Build history of the part. All positions in model axes, mm. Coordinates: 2 decimals unless noted, no trailing zeros. Order: outer loops, then holes, each group sorted by start corner. A loop starts at its lowest first (then second) coordinate and runs counter-clockwise, first axis right, second up. Notation, with made-up numbers: (86.25, 13) - (123.25, 13) arc R24 ccw to (123.25, 31) - close; hole circle Ø4 at (-11, 39). An arc over 180 degrees is marked (long way). Write each question's results on one line, items separated by ' | '.
from build123d import *

# Parameters (mm, degrees)
SKETCH1_W           = 63.5
SKETCH1_H           = 101.6
SKETCH1_R           = 20.955
SKETCH1_R_2         = 3.175
BOSS_EXTRUDE1_DEPTH = 4.7625
CHAMFER1_SIZE       = 3.8862
CHAMFER1_SIZE2      = 3.378222121


with BuildPart() as part:
    # Sketch1 → Boss-Extrude1 (new body)
    with BuildSketch(Plane(origin=(0, 0, 0), x_dir=(1, 0, 0), z_dir=(0, 1, 0))):
        with Locations((31.75, 50.8)):
            Rectangle(SKETCH1_W, SKETCH1_H)
        with Locations((31.75, 50.8)):
            Circle(SKETCH1_R, mode=Mode.SUBTRACT)
        with Locations((9.525, 92.075)):
            Circle(SKETCH1_R_2, mode=Mode.SUBTRACT)
        with Locations((53.975, 92.075)):
            Circle(SKETCH1_R_2, mode=Mode.SUBTRACT)
        with Locations((53.975, 9.525)):
            Circle(SKETCH1_R_2, mode=Mode.SUBTRACT)
        with Locations((9.525, 9.525)):
            Circle(SKETCH1_R_2, mode=Mode.SUBTRACT)
    extrude(amount=BOSS_EXTRUDE1_DEPTH)

    # Chamfer1
    chamfer1_edges = [part.edges().sort_by_distance(p)[0] for p in [
        (6.35, 4.7625, -92.075),
        (50.8, 4.7625, -92.075),
        (50.8, 4.7625, -9.525),
        (6.35, 4.7625, -9.525),
    ]]
    chamfer1_side = [part.faces().sort_by_distance(p)[0] for p in [
        (31.75, 4.7625, -1.198115604),
    ]]
    chamfer(chamfer1_edges, length=CHAMFER1_SIZE, length2=CHAMFER1_SIZE2, reference=chamfer1_side[0])


solid = part.part
1. Band-saw the part on C-C on y = 3.55. Give the cut face in (x, z) (3 decimals), then the cut area to 3 significant figures.
Solved:
outline: (0, -101.6) - (63.5, -101.6) - (63.5, 0) - (0, 0) - close; hole circle Ø11.333 at (9.525, -92.075); hole circle Ø11.333 at (9.525, -9.525); hole circle Ø41.91 at (31.75, -50.8); hole circle Ø11.333 at (53.975, -92.075); hole circle Ø11.333 at (53.975, -9.525) | area: 4,670 mm2
2. Two-plate mould, pull along X, no slides. Class faces 1 (the face through (10, 0, -52)), 2 (the face through (63.5, 2, -50)), 3 (the face through (12.632, 1.548, -8.237)): +X half, -X half, draft (parallel to the pull), parting line (faces both ways), or undercut.
Solved:
face 1: draft | face 2: +X half | face 3: undercut
3. Band-saw the part on B-B on z = -50.8. Give the cut face in (x, y) (1 decimal), then the cut area to 3 significant figures.
Solved:
outline: (0, 0) - (10.8, 0) - (10.8, 4.8) - (0, 4.8) - close; (52.7, 0) - (63.5, 0) - (63.5, 4.8) - (52.7, 4.8) - close | area: 103 mm2
4. Probe line 1 (X direction, y = 2.85, z = -8); line 2 (Z direction, x = 54.5, y = 4.5); line 3 (Z direction, x = 7.5, y = 1.15). List the from-to ranges inside material, lowest first.
Solved:
line 1: x = 0 to 4.91, 14.14 to 49.36, 58.59 to 63.5 | line 2: z = -101.6 to -98.81, -85.34 to -16.26, -2.79 to 0 | line 3: z = -101.6 to -94.52, -89.63 to -11.97, -7.08 to 0
5. Band-saw the part on A-A on x = 31.75. Give the cut face in (y, z) (1 decimal).
Solved:
outline: (0, -101.6) - (4.8, -101.6) - (4.8, -71.8) - (0, -71.8) - close; (0, -29.8) - (4.8, -29.8) - (4.8, 0) - (0, 0) - close
